Autodesk Inventor part; units mm, degrees
ref_plane "YZ Plane" through (0, 0, 0) normal (1, 0, 0) x (0, 1, 0)
ref_plane "XZ Plane" through (0, 0, 0) normal (0, 1, 0) x (-1, 0, 0)
ref_plane "XY Plane" through (0, 0, 0) normal (0, 0, 1) x (1, 0, 0)
sketch "Sketch1" plane through (0, 0, 0) normal (0, 0, 1) x (1, 0, 0)
  line L0 (0, 0) -> (304.8, 0)
  line L1 (304.8, 0) -> (304.8, 304.8)
  line L2 (304.8, 304.8) -> (0, 304.8)
  line L3 (0, 304.8) -> (0, 0)
  circle A0 centre (152.4, 152.4) radius 114.3
  circle A1 centre (6.35, 298.45) radius 0.9922
  circle A2 centre (298.45, 298.45) radius 0.9922
  circle A3 centre (298.45, 6.35) radius 0.9922
  circle A4 centre (6.35, 6.35) radius 0.9922
  circle A5 centre (6.35, 152.4) radius 0.9922
  circle A6 centre (298.45, 152.4) radius 0.9922
  circle A7 centre (152.4, 298.45) radius 0.9922
  circle A8 centre (152.4, 6.35) radius 0.9922
  point P0 (304.8, 152.4)
  point P1 (152.4, 304.8)
  dimension "d0" = 304.8
  dimension "d1" = 228.6
  dimension "d6" = 1.9844
  dimension "d7" = 6.35
  dimension "d8" = 6.35
  dimension "d10" = 6.35
  dimension "d11" = 6.35
extrude "Extrusion1" add sketch "Sketch1" against normal blind 12.7 contours L3 L2 L1 L0 | A1 | A2 | A3 | A4 | A5 | A6 | A7 | A8
hole "Hole1" at (6.35, 298.45, 0) at (298.45, 298.45, 0) at (298.45, 6.35, 0) at (6.35, 6.35, 0) at (152.4, 298.45, 0) at (152.4, 6.35, 0) at (298.45, 152.4, 0) at (6.35, 152.4, 0) direction (0, 0, -1) diameter 3.2766 end through all countersink diameter 5.715 countersink angle 82
equation "\"d10\" = d7"
equation "\"d11\" = d8"
properties material "MDF Medium Density Fiberboard"
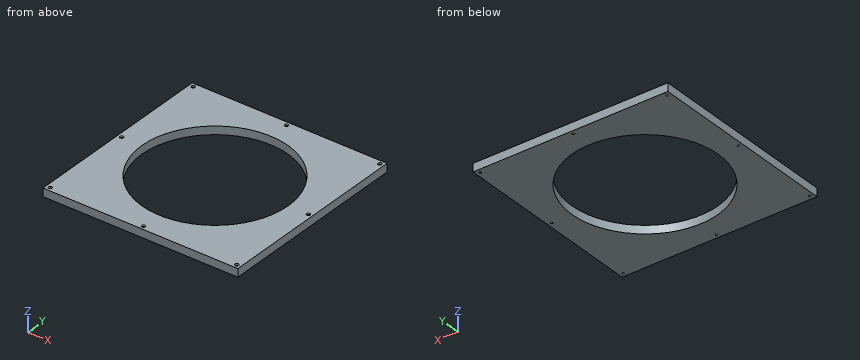
For this review, take the finished solid that the model builds, in its own axes (mm). Round coordinates to 2 decimals unless told otherwise and drop trailing zeros. Order: outer loops, then holes, each group sorted by start corner. A loop starts at its lowest first (then second) coordinate and runs counter-clockwise, first axis right, second up. Notation, with made-up numbers: (-32.5, 59) -> (-2.5, 59) arc R21 cw to (-2.5, 72) -> close; hole circle Ø11 at (79.5, 40). An arc over 180 degrees is marked (long way). Write item = value, one per line. Start each with the question number.
1) Insertion check: pin 1 (2.5 mm diameter, centred on x = 6.35, y = 298.45, fed in from -Z); pin 2 (4 mm diameter, centred on x = 298.45, y = 298.45, fed in from +Z); pin 3 (4.5 mm diameter, centred on x = 6.35, y = 6.35, fed in from +Z). Each pin has a flat end and moves straight along its axis. Give the tip position at first contact, or say it passes through.
2) Take a section at B-B on y = 97.5. State the section outline as (x, z) points.
3) Take a section at A-A on z = -7.75. Count the separate pieces of the cut face and the enclosed holes in it, plus the area to 3 significant figures.
4) To check wall thickness, follow line 1 (Y direction, x = 6.35, z = -6.75); line 2 (Y direction, x = 152.4, z = -9.5). State the ranges of each line that lie inside material, in increasing order. Write a range as from..to.
5) Take a section at C-C on x = 189.5. State the section outline as (y, z) points.
Verdict:
q1.pin_1 = through
q1.pin_2 = -0.99
q1.pin_3 = -0.7
q2.outline = (0, -12.7) -> (52.15, -12.7) -> (52.15, 0) -> (0, 0) -> close; (252.65, -12.7) -> (304.8, -12.7) -> (304.8, 0) -> (252.65, 0) -> close
q3.separate_pieces = 1
q3.enclosed_holes = 9
q3.area = 51,800 mm2
q4.line_1 = 0..4.71, 7.99..150.76, 154.04..296.81, 300.09..304.8
q4.line_2 = 0..4.71, 7.99..38.1, 266.7..296.81, 300.09..304.8
q5.outline = (0, -12.7) -> (44.29, -12.7) -> (44.29, 0) -> (0, 0) -> close; (260.51, -12.7) -> (304.8, -12.7) -> (304.8, 0) -> (260.51, 0) -> close
